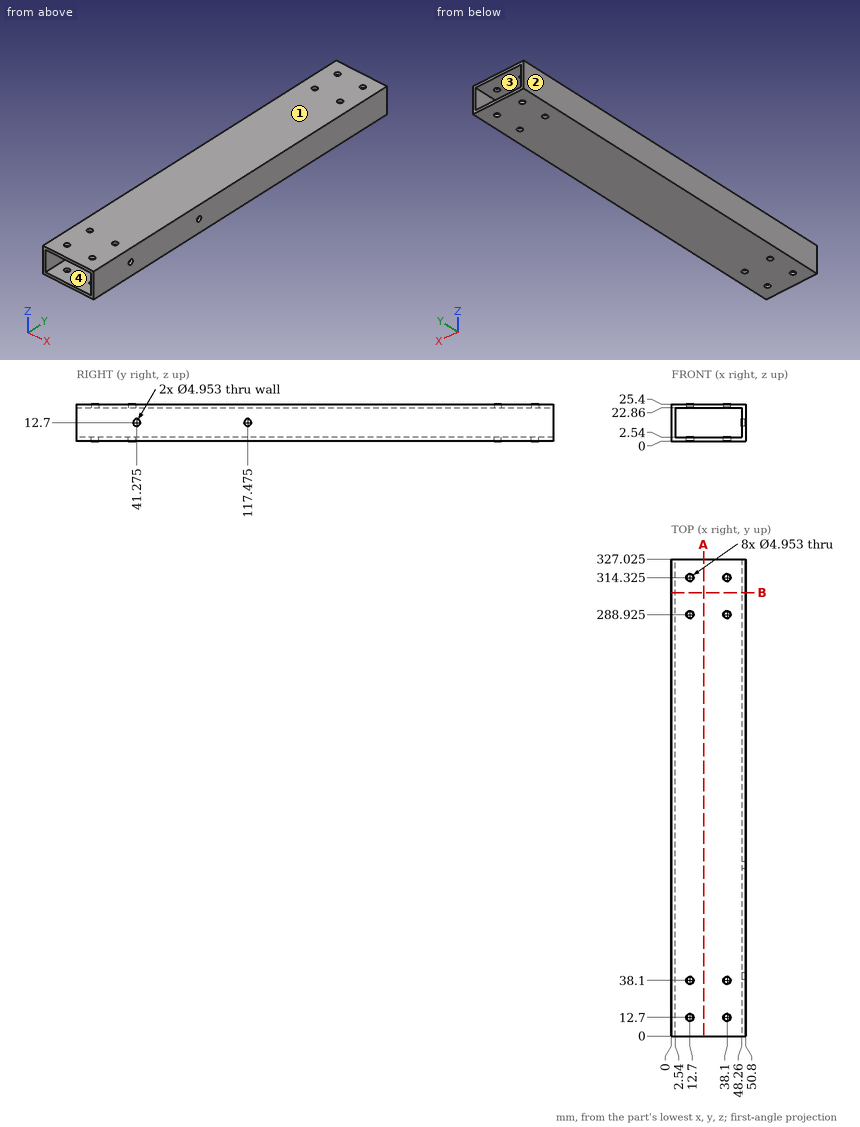
Answer from the drawing. Dimensions are ordinates in mm from the lowest x, y and z of the part. Coordinates: 2 decimals unless noted, no trailing zeros. Order: outer loops, then holes, each group sorted by start corner. A loop starts at its lowest first (then second) coordinate and runs counter-clockwise, first axis right, second up. Notation, with made-up numbers: (47, -3.5) - (100, -3.5) arc R29 cw to (100, 31.5) - close; hole circle Ø6 at (65.5, 79.25). An arc over 180 degrees is marked (long way). Put each result on its own line as item: value. Start each with the question number.
1) For a pull along Z with two mould halves and no side action, classify the marked faces 1, 2, 3 and 4 as released by +Z, released by -Z, zero draft, split by the parting line, or undercut.
2) Find section B-B (y = 304). Give the vertices of the cut face in (x, z).
3) Find section A-A (x = 22). Give the vertices of the cut face in (y, z) (3 decimals).
4) Flat-ended cylindrical pins translate along their axes: pin 1 (3 mm diameter, centred on x = 38.1, y = 12.7, fed in from +Z); pin 2 (5 mm diameter, centred on x = 42.5, z = 20.5, fed in from +Y) (3 decimals). Find the tip coordinate at first contact, or state that the pin passes through.
5) Find the intervals of material crossed by line 1 (Y direction, x = 12.7, z = 1.45) (1 decimal); line 2 (Y direction, x = 49, z = 12.7) (1 decimal); line 3 (X direction, y = 12.7, z = 0.9), in increasing order. Write a range as from..to.
Results list:
1. face 1: released by +Z
1. face 2: zero draft
1. face 3: undercut
1. face 4: undercut
2. outline: (0, 0) - (50.8, 0) - (50.8, 25.4) - (0, 25.4) - close; hole (2.54, 2.54) - (48.26, 2.54) - (48.26, 22.86) - (2.54, 22.86) - close
3. outline: (0, 0) - (327.025, 0) - (327.025, 2.54) - (0, 2.54) - close; (0, 22.86) - (327.025, 22.86) - (327.025, 25.4) - (0, 25.4) - close
4. pin 1: passes through
4. pin 2: stops at y = 327.025
5. line 1: y = 0..10.2, 15.2..35.6, 40.6..286.4, 291.4..311.8, 316.8..327
5. line 2: y = 0..38.8, 43.8..115, 120..327
5. line 3: x = 0..10.22, 15.18..35.62, 40.58..50.8
